Read the model definition and answer for the solid it produces. Units are mm, in the model's axes. A direction names the side the tool comes from. Give positions to 0.01 mm unless a question says otherwise; leave off trailing zeros. Write each loop counter-clockwise with the first axis right and the second up, starting at its lowest first coordinate (ties: lowest second). Pieces come first, ordered by that corner, then holes.
```python
from build123d import *

# Parameters (mm, degrees)
CUT_EXTRUDE1_DEPTH = 1


with BuildPart() as part:
    # Sketch1 → Revolve5 (revolve)
    with BuildSketch(Plane.XY, mode=Mode.PRIVATE) as revolve5_sk:
        Polygon((6.5, 0), (3, -5), (3, -18), (0, -19.732050808), (0, 0), align=None)
    revolve(revolve5_sk.sketch.rotate(Axis((0, 0, 0), (0, 1, 0)), 90), axis=Axis((0, 0, 0), (0, 1, 0)))

    # Sketch2 → Cut-Extrude1 (cut)
    with BuildSketch(Plane(origin=(0, 0, 0), x_dir=(1, 0, 0), z_dir=(0, 1, 0))):
        with BuildLine():
            Line((0, -6.5), (0, 6.5))
            ThreePointArc((0, 6.5), (-0.501494825, 6.480625197), (-1, 6.422616289))
            Line((-1, 6.422616289), (-1, -6.422616289))
            ThreePointArc((-1, -6.422616289), (-0.501494825, -6.480625197), (0, -6.5))
        make_face()
        with BuildLine():
            ThreePointArc((1, 6.422616289), (0.501494825, 6.480625197), (0, 6.5))
            Line((0, 6.5), (0, -6.5))
            ThreePointArc((0, -6.5), (0.501494825, -6.480625197), (1, -6.422616289))
            Line((1, -6.422616289), (1, 6.422616289))
        make_face()
    extrude(amount=-CUT_EXTRUDE1_DEPTH, mode=Mode.SUBTRACT)


solid = part.part
```
Item 1: Find the intervals of material crossed by line 1 along Y through (x, z) = (1.25, -1.5); line 2 along X through (y, z) = (-7.5, -1.25); line 3 along Y through (x, z) = (-3, 1.5), in increasing order.
Result set:
line 1: y = -18.6 to 0
line 2: x = -2.73 to 2.73
line 3: y = -4.49 to 0
Item 2: Each of these flat-tipped pins is pushed along its axis until it touches: pin 1 Ø1 at (x, y) = (-3, -4) entering from -Z; pin 2 Ø4 at (y, z) = (-11.5, 2.5) entering from -X; pin 3 Ø6 at (x, z) = (5, 5) entering from -Y. Where does it stop, or does it pass through?
Result set:
pin 1: stops at z = -2.93
pin 2: stops at x = -2.96
pin 3: stops at y = -3.47
Item 3: Which of the six approach directions +Z, -Z, +X, -X, +Y, -Y give full straight-line access (tool end or side, diameter ignored) to faces 4 (the flat face through (-3, 0, 0)), 5 (the flat face through (0, -1, 0)), 6 (the cylindrical face through (-0.9, -11.59, -2.86))?
Result set:
face 4: +Z, -Z, +X, -X, +Y
face 5: +Z, -Z, +Y
face 6: -Y
Item 4: Determine the mould class of faces 1 (the flat face through (3, 0, 0)), 2 (the conical face through (-0.95, -4.76, -3.02)), 3 (the flat face through (-1, -0.5, -0.1)) for opening direction X: pulls with the +X half, pulls with the -X half, needs draft (parallel to the pull), parting line crosses it, or undercut.
Result set:
face 1: needs draft
face 2: parting line crosses it
face 3: undercut
Item 5: Section A-A (y = -6.5) is taken. Write down the section's boundary in (x, z).
Result set:
outline: circle Ø6 at (0, 0)
